```python
from build123d import *

# Parameters (mm, degrees)
BOSS_EXTRUDE1_DEPTH = 25.5
SKETCH3_R           = 4
CUT_EXTRUDE1_DEPTH  = 39.320882036
SKETCH3_4_R         = 6.5
SKETCH3_4_R_2       = 4
CUT_EXTRUDE2_DEPTH  = 6
SKETCH9_R           = 1.0922
CUT_EXTRUDE3_DEPTH  = 41.712283159
FILLET1_R           = 10
FILLET2_R           = 5
FILLET4_R           = 2
CHAMFER1_SIZE       = 1


with BuildPart() as part:
    # Sketch1 → Boss-Extrude1 (new, symmetric)
    with BuildSketch(Plane.XY):
        Polygon((-22.2, -8.5), (3.2, -8.5), (3.2, 1.5), (26.8, 1.5), (26.8, 8.5), (-3.2, 8.5), (-3.2, 1.5), (-22.2, 1.5), align=None)
    extrude(amount=BOSS_EXTRUDE1_DEPTH, both=True)

    # Sketch3 → Cut-Extrude1 (cut, through all)
    with BuildSketch(Plane(origin=(0, 1.5, 0), x_dir=(1, 0, 0), z_dir=(0, 1, 0))):
        with Locations(Location((-9.7, -12.7, 0), (0, 0, 180))):
            Circle(SKETCH3_R)
    cut_extrude1 = extrude(amount=-CUT_EXTRUDE1_DEPTH, mode=Mode.SUBTRACT)

    # Sketch3<4> → Cut-Extrude2 (cut)
    with BuildSketch(Plane(origin=(0, 1.5, 0), x_dir=(1, 0, 0), z_dir=(0, 1, 0))):
        with Locations(Location((-9.7, -12.7, 0), (0, 0, 180))):
            Circle(SKETCH3_4_R)
        with Locations(Location((-9.7, -12.7, 0), (0, 0, 180))):
            Circle(SKETCH3_4_R_2, mode=Mode.SUBTRACT)
    cut_extrude2 = extrude(amount=-CUT_EXTRUDE2_DEPTH, mode=Mode.SUBTRACT)

    # Mirror1: Cut-Extrude1, Cut-Extrude2 across plane
    add(cut_extrude1.mirror(Plane.XY), mode=Mode.SUBTRACT)
    add(cut_extrude2.mirror(Plane.XY), mode=Mode.SUBTRACT)

    # Sketch9 → Cut-Extrude3 (cut, through all)
    with BuildSketch(Plane(origin=(0, 8.5, 0), x_dir=(1, 0, 0), z_dir=(0, 1, 0))):
        with Locations(Location((10.4078, 11.1, 0), (0, 0, 180))):
            Circle(SKETCH9_R)
        with Locations(Location((20.7078, -11.1, 0), (0, 0, 180))):
            Circle(SKETCH9_R)
    extrude(amount=-CUT_EXTRUDE3_DEPTH, mode=Mode.SUBTRACT)

    # Fillet1
    # the kernel refuses this fillet: 10 mm, written as the material it adds along each edge
    with BuildSketch(Plane(origin=(-3.2, 1.5, 25.5), x_dir=(0, 1, 0), z_dir=(0, 0, -1))) as fillet1_piece_1_section:
        with BuildLine():
            CenterArc((10, -9.539392014), FILLET1_R, 107.457603124, 72.542396876)
            Line((0, -9.539392014), (0, 0))
            Line((0, 0), (7, 0))
        make_face()
    fillet1_piece_1 = extrude(amount=12.8, mode=Mode.PRIVATE)
    fillet1_piece_1 = fillet1_piece_1 - Plane(origin=(-9.7, 1.5, 12.7), x_dir=(-1, 0, 0), z_dir=(0, 1, 0)) * Cylinder(6.5, 64, mode=Mode.PRIVATE)
    add(fillet1_piece_1)
    with BuildSketch(Plane(origin=(-3.2, 1.5, -12.700000035), x_dir=(0, 1, 0), z_dir=(0, 0, -1))) as fillet1_piece_2_section:
        with BuildLine():
            CenterArc((10, -9.539392014), FILLET1_R, 107.457603124, 72.542396876)
            Line((0, -9.539392014), (0, 0))
            Line((0, 0), (7, 0))
        make_face()
    fillet1_piece_2 = extrude(amount=12.799999965, mode=Mode.PRIVATE)
    fillet1_piece_2 = fillet1_piece_2 - Plane(origin=(-9.7, 1.5, -12.7), x_dir=(-1, 0, 0), z_dir=(0, 1, 0)) * Cylinder(6.5, 64, mode=Mode.PRIVATE)
    add(fillet1_piece_2)
    with BuildSketch(Plane(origin=(-3.2, 1.5, 12.7), x_dir=(0, 1, 0), z_dir=(0, 0, -1))) as fillet1_piece_3_section:
        with BuildLine():
            CenterArc((10, -9.539392014), FILLET1_R, 107.457603124, 72.542396876)
            Line((0, -9.539392014), (0, 0))
            Line((0, 0), (7, 0))
        make_face()
    fillet1_piece_3 = extrude(amount=25.400000035, mode=Mode.PRIVATE)
    fillet1_piece_3 = fillet1_piece_3 - Plane(origin=(-9.7, 1.5, -12.7), x_dir=(-1, 0, 0), z_dir=(0, 1, 0)) * Cylinder(6.5, 89, mode=Mode.PRIVATE)
    fillet1_piece_3 = fillet1_piece_3 - Plane(origin=(-9.7, 1.5, 12.7), x_dir=(-1, 0, 0), z_dir=(0, 1, 0)) * Cylinder(6.5, 89, mode=Mode.PRIVATE)
    add(fillet1_piece_3)

    # Fillet2
    # the kernel refuses this fillet: 5 mm, written as the material it adds along each edge
    with BuildSketch(Plane(origin=(3.2, 1.5, -25.5), x_dir=(0, -1, 0), z_dir=(0, 0, 1))) as fillet2_piece_1:
        with BuildLine():
            CenterArc((FILLET2_R, FILLET2_R), FILLET2_R, 180, 90)
            Line((0, FILLET2_R), (0, 0))
            Line((0, 0), (FILLET2_R, 0))
        make_face()
    extrude(amount=51)
    # the kernel refuses this fillet: 5 mm, written as the material it takes off along each edge
    with BuildSketch(Plane(origin=(-3.2, 8.5, -33.372963816), x_dir=(1, 0, 0), z_dir=(0, 0, 1))) as fillet2_2_piece_1:
        with BuildLine():
            CenterArc((3.149185526, -5), FILLET2_R, 90, 57.769047364)
            ThreePointArc((-1.080340321, -2.333333333), (-0.464861443, -1.201534828), (0, 0))
            Line((0, 0), (3.149185526, 0))
        make_face()
    extrude(amount=20.67296378, mode=Mode.SUBTRACT)
    with BuildSketch(Plane(origin=(-22.2, 1.5, 38), x_dir=(1, 0, 0), z_dir=(0, 0, -1))) as fillet2_2_piece_2:
        with BuildLine():
            CenterArc((FILLET2_R, FILLET2_R), FILLET2_R, 180, 90)
            Line((0, FILLET2_R), (0, 0))
            Line((0, 0), (FILLET2_R, 0))
        make_face()
    extrude(amount=76, mode=Mode.SUBTRACT)
    with BuildSketch(Plane(origin=(-3.2, 8.5, -12.700000035), x_dir=(-0.42015348282673015, -0.9074530571156663, 0), z_dir=(0, 0, 1))) as fillet2_2_piece_3:
        with BuildLine():
            CenterArc((3.214124019, 4.958505447), FILLET2_R, 204.84427788, 57.769047364)
            Line((-1.323141267, 2.857738033), (0, 0))
            ThreePointArc((0, 0), (1.285649607, 0.082989105), (2.571299215, 0))
        make_face()
    extrude(amount=25.400000035, mode=Mode.SUBTRACT)
    with BuildSketch(Plane(origin=(-3.2, 8.5, 12.7), x_dir=(1, 0, 0), z_dir=(0, 0, 1))) as fillet2_2_piece_4:
        with BuildLine():
            CenterArc((3.149185526, -5), FILLET2_R, 90, 57.769047364)
            ThreePointArc((-1.080340321, -2.333333333), (-0.464861443, -1.201534828), (0, 0))
            Line((0, 0), (3.149185526, 0))
        make_face()
    extrude(amount=20.672963816, mode=Mode.SUBTRACT)

    # Fillet4
    fillet4_edges = [part.edges().sort_by_distance(p)[0] for p in [
        (26.8, 8.5, 0),
        (26.8, 1.5, 0),
    ]]
    fillet(fillet4_edges, radius=FILLET4_R)

    # Chamfer1
    chamfer1_edges = [part.edges().sort_by_distance(p)[0] for p in [
        (12.374592763, 8.5, 25.5),
        (12.374592763, 8.5, -25.5),
        (26.8, 5, -25.5),
        (26.214213562, 2.085786438, -25.5),
        (26.214213562, 7.914213562, -25.5),
        (26.8, 5, 25.5),
        (26.214213562, 2.085786438, 25.5),
        (26.214213562, 7.914213562, 25.5),
        (3.2, -6, -25.5),
        (-9.5, -8.5, -25.5),
        (3.2, -6, 25.5),
        (-14.969696007, 1.5, -25.5),
        (-14.969696007, 1.5, 25.5),
        (-7.908933099, 2.744049642, -25.5),
        (-7.908933099, 2.744049642, 25.5),
        (-22.2, -6, 25.5),
        (16.5, 1.5, 25.5),
        (-20.735533906, 0.035533906, 25.5),
        (-2.466043931, 7.877975179, 25.5),
        (-22.2, -6, -25.5),
        (16.5, 1.5, -25.5),
        (-20.735533906, 0.035533906, -25.5),
        (-2.466043931, 7.877975179, -25.5),
        (4.664466094, 0.035533906, -25.5),
        (4.664466094, 0.035533906, 25.5),
        (-9.5, -8.5, 25.5),
    ]]
    chamfer(chamfer1_edges, length=CHAMFER1_SIZE)


solid = part.part
```
For this review, take the finished solid that the model builds, in its own axes (mm). A direction names the side the tool comes from. Round coordinates to 2 decimals unless told otherwise and drop trailing zeros. Loops run counter-clockwise (first coordinate to the right, second up) from the corner with the lowest first, then second, coordinate; pieces in that order, holes last.
(1) We need section B-B (z = -11.1). Give the boundary of the cut face in (x, y), plus the area to 3 significant figures.
Returned:
outline: (-22.2, -8.5) - (-13.37, -8.5) - (-13.37, -4.5) - (-16, -4.5) - (-16, 1.5) - (-17.2, 1.5) arc R5 ccw to (-22.2, -3.5) - close; (-6.03, -8.5) - (3.2, -8.5) - (3.2, -3.5) arc R5 cw to (8.2, 1.5) - (9.32, 1.5) - (9.32, 8.5) - (-0.05, 8.5) arc R5 ccw to (-3.4, 7.21) - (-3.4, -4.5) - (-6.03, -4.5) - close; (11.5, 1.5) - (24.8, 1.5) arc R2 ccw to (26.8, 3.5) - (26.8, 6.5) arc R2 ccw to (24.8, 8.5) - (11.5, 8.5) - close
area: 342 mm2
(2) We need section C-C (y = -2.25). State how many separate pieces and enclosed holes the cut face has, plus the area to 3 significant figures.
Returned:
separate pieces: 1
enclosed holes: 2
area: 1,030 mm2
(3) Clearance check with flat-ended pins moving along their axes: P1, Ø5, axis at x = -14, z = -2.5, coming from the +Y side; P2, Ø10.5, axis at x = -10, z = 16, coming from the +Y side; P3, Ø4, axis at x = -13, z = -13, coming from the +Y side. State where each tip first meets the part, or that it passes through.
Returned:
P1: stops at y = 1.58
P2: stops at y = 5.35
P3: stops at y = -4.5
(4) Mouldability with a two-part tool opening along Z and no side actions: class faces 1 (the cylindrical face through (-11.546, -6.472, 9.151)), 2 (the cylindrical face through (26.2, 2.07, 0.34)), 3 (the conical face through (-20.196, -0.437, 25.215)) as released by +Z, released by -Z, zero draft, split by the parting line, or undercut.
Returned:
face 1: undercut
face 2: zero draft
face 3: released by +Z
(5) We need section A-A (z = 21). Give the boundary of the cut face in (x, y), plus the area to 3 significant figures.
Returned:
outline: (-22.2, -8.5) - (3.2, -8.5) - (3.2, -3.5) arc R5 cw to (8.2, 1.5) - (24.8, 1.5) arc R2 ccw to (26.8, 3.5) - (26.8, 6.5) arc R2 ccw to (24.8, 8.5) - (-0.05, 8.5) arc R5 ccw to (-4.28, 6.17) arc R10 cw to (-12.74, 1.5) - (-17.2, 1.5) arc R5 ccw to (-22.2, -3.5) - close
area: 479 mm2
(6) Wall thickness on line 1 along Z through (x, y) = (-9.7, -5.6); line 2 along X through (y, z) = (-7, -12.7); line 3 along Z through (x, y) = (-9.7, 1.25): over which ranges is each line inside the solid? List them lowest first.
Returned:
line 1: z = -25.5 to -16.7, -8.7 to 8.7, 16.7 to 25.5
line 2: x = -22.2 to -13.7, -5.7 to 3.2
line 3: z = -25.19 to -19.2, -6.2 to 6.2, 19.2 to 25.19
(7) Tool access review of faces 4 (the flat face through (-10, -4.5, 8)), 5 (the flat face through (16, 1.5, 0)), 6 (the flat face through (-15, 1.5, 0)), 7 (the flat face through (-10, -8.5, 0)): name each direction out of +Z, -Z, +X, -X, +Y, -Y from which nothing blocks a thin tool from reaching the whole face with its end or side.
Returned:
face 4: +Y
face 5: +Z, -Z, +X, -Y
face 6: +Z, -Z, -X, +Y
face 7: +Z, -Z, +X, -X, -Y
